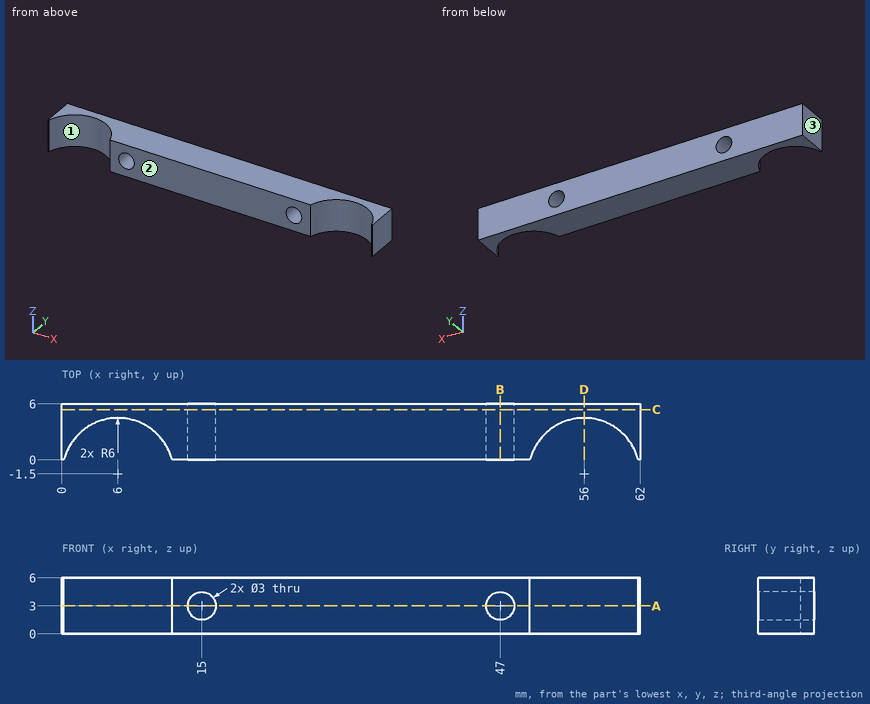
Geometry check sheet. Reference: drawing and pictorial views, mm from the part's lowest x, y, z. Round coordinates to 2 decimals unless told otherwise and drop trailing zeros. Loops run counter-clockwise (first coordinate to the right, second up) from the corner with the lowest first, then second, coordinate; pieces in that order, holes last. Notation, with made-up numbers: (78, -27.5) -> (92, -27.5) arc R19 cw to (92, 1.5) -> close; hole circle Ø6 at (68, 34). An arc over 180 degrees is marked (long way). Answer as a JSON object with one key per item and string values. Group by question number.
Item 1: Thickness scan on line 1 along X through (y, z) = (5.4, 3.25); line 2 along X through (y, z) = (1.2, 3); line 3 along X through (y, z) = (3.5, 3). Record the ranges inside material, lowest first.
Item 2: Release check for a two-part mould opening along X. For the marked faces 1, 2 and 3 record: pulls with the +X half, pulls with the -X half, needs draft (parallel to the pull), parting line crosses it, or undercut.
Item 3: Cross-section at A-A, the plane z = 3. Record the cut outline in (x, y), plus the area to 3 significant figures.
Item 4: Cross-section at D-D, the plane x = 56. Record the cut outline in (y, z).
Item 5: Cross-section at B-B, the plane x = 47. Record the cut outline in (y, z), plus the area to 3 significant figures.
Item 6: Cross-section at C-C, the plane y = 5.4. Record the cut outline in (x, z).
Determined:
{
 "1": {"line 1": "x = 0 to 13.52, 16.48 to 45.52, 48.48 to 62", "line 2": "x = 0 to 0.64, 11.36 to 13.5, 16.5 to 45.5, 48.5 to 50.64, 61.36 to 62", "line 3": "x = 0 to 2.68, 9.32 to 13.5, 16.5 to 45.5, 48.5 to 52.68, 59.32 to 62"},
 "2": {"face 1": "undercut", "face 2": "needs draft", "face 3": "pulls with the -X half"},
 "3": {"outline": "(0, 0) -> (0.19, 0) arc R6 cw to (11.81, 0) -> (13.5, 0) -> (13.5, 6) -> (0, 6) -> close; (16.5, 0) -> (45.5, 0) -> (45.5, 6) -> (16.5, 6) -> close; (48.5, 0) -> (50.19, 0) arc R6 cw to (61.81, 0) -> (62, 0) -> (62, 6) -> (48.5, 6) -> close", "area": "259 mm²"},
 "4": {"outline": "(4.5, 0) -> (6, 0) -> (6, 6) -> (4.5, 6) -> close"},
 "5": {"outline": "(0, 0) -> (6, 0) -> (6, 1.5) -> (0, 1.5) -> close; (0, 4.5) -> (6, 4.5) -> (6, 6) -> (0, 6) -> close", "area": "18.0 mm²"},
 "6": {"outline": "(0, 0) -> (62, 0) -> (62, 6) -> (0, 6) -> close; hole circle Ø3 at (15, 3); hole circle Ø3 at (47, 3)"}
}
